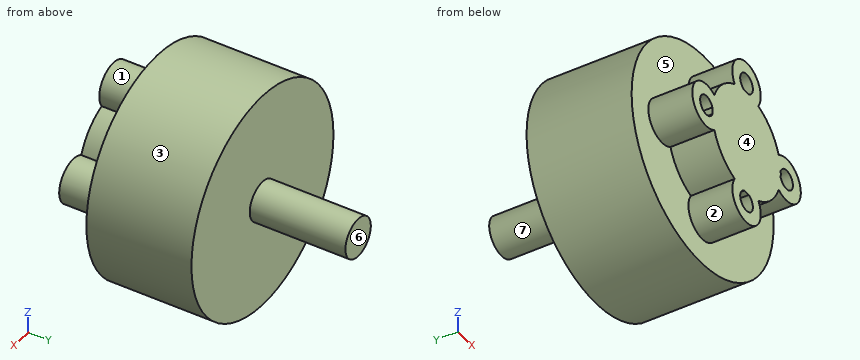
```python
from build123d import *

# Parameters (mm, degrees)
SKETCH1_R           = 14
BOSS_EXTRUDE1_DEPTH = 13.4
SKETCH2_R           = 2.5
BOSS_EXTRUDE2_DEPTH = 12.2
SKETCH3_R           = 6.75
BOSS_EXTRUDE3_DEPTH = 5.6


with BuildPart() as part:
    # Sketch1 → Boss-Extrude1 (new body)
    with BuildSketch(Plane(origin=(0, 0, 0), x_dir=(1, 0, 0), z_dir=(0, 1, 0))):
        Circle(SKETCH1_R)
    extrude(amount=BOSS_EXTRUDE1_DEPTH)

    # Sketch2 → Boss-Extrude2 (add)
    with BuildSketch(Plane(origin=(0, 13.4, 0), x_dir=(1, 0, 0), z_dir=(0, 1, 0))):
        Circle(SKETCH2_R)
    extrude(amount=BOSS_EXTRUDE2_DEPTH)

    # Sketch3 → Boss-Extrude3 (add)
    with BuildSketch(Plane.XZ):
        Circle(SKETCH3_R)
        with BuildLine():
            ThreePointArc((-6.734810127, 0.452584311), (-6.602756441, 1.402179513), (-6.3375, 2.323487411))
            ThreePointArc((-6.3375, 2.323487411), (-10.7, 0), (-6.3375, -2.323487411))
            ThreePointArc((-6.3375, -2.323487411), (-6.602756441, -1.402179513), (-6.734810127, -0.452584311))
            ThreePointArc((-6.734810127, -0.452584311), (-9.15, 0), (-6.734810127, 0.452584311))
        make_face()
        with BuildLine():
            ThreePointArc((0.452584311, 6.734810127), (1.402179513, 6.602756441), (2.323487411, 6.3375))
            ThreePointArc((2.323487411, 6.3375), (0, 10.7), (-2.323487411, 6.3375))
            ThreePointArc((-2.323487411, 6.3375), (-1.402179513, 6.602756441), (-0.452584311, 6.734810127))
            ThreePointArc((-0.452584311, 6.734810127), (0, 9.15), (0.452584311, 6.734810127))
        make_face()
        with BuildLine():
            ThreePointArc((-2.323487411, -6.3375), (0, -10.7), (2.323487411, -6.3375))
            ThreePointArc((2.323487411, -6.3375), (1.402179513, -6.602756441), (0.452584311, -6.734810127))
            ThreePointArc((0.452584311, -6.734810127), (0, -9.15), (-0.452584311, -6.734810127))
            ThreePointArc((-0.452584311, -6.734810127), (-1.402179513, -6.602756441), (-2.323487411, -6.3375))
        make_face()
        with BuildLine():
            ThreePointArc((6.3375, 2.323487411), (6.602756441, 1.402179513), (6.734810127, 0.452584311))
            ThreePointArc((6.734810127, 0.452584311), (9.15, 0), (6.734810127, -0.452584311))
            ThreePointArc((6.734810127, -0.452584311), (6.602756441, -1.402179513), (6.3375, -2.323487411))
            ThreePointArc((6.3375, -2.323487411), (10.7, 0), (6.3375, 2.323487411))
        make_face()
    extrude(amount=BOSS_EXTRUDE3_DEPTH)


solid = part.part
```
Can you work these out from the model? Positions are in its coordinate system, mm. Face numbers are marked on the shaded views. A direction names the side the tool comes from. Coordinates: 2 decimals unless noted, no trailing zeros. Write each loop counter-clockwise with the first axis right and the second up, starting at its lowest first coordinate (ties: lowest second). Pieces come first, ordered by that corner, then holes. Notation, with made-up numbers: M -20.75,43 L 13.25,43 A14 cw 13.25,48 Z; hole C 39.25,8.5 d1. An arc over 180 degrees is marked long. Write item = value, one per line. Start each with the question number.
Q1. If we section it at B-B, the plane x = 0: Write out the boundary of the cut face in (y, z).
Q2. If I drill on L1, parallel to X at y = -3.05, z = 0; L2, parallel to X at y = -2.95, z = 7.9, over which ranges is the centre line in solid material (lowest first)? Write a range as [from, to].
Q3. On a 3-axis mill with a long thin cutter (end or side, diameter ignored), from which of +Z, -Z, +X, -X, +Y, -Y can I reach the whole of each face in a straight line? I mean the marked faces 5, 6 and 7. Say none if no direction works.
Q4. If we section it at A-A, the plane z = 0: Write out the boundary of the cut face in (x, y), then the cut area to 3 significant figures.
Q5. Thinking about a two-plate mould opening in Z: for the marked faces 1, 2, 3 and 4, which applies, released by +Z, released by -Z, zero draft, split by the parting line, or undercut?
Q6. I'm going to push flat-ended pins straight in: pin 1 (12 mm diameter, centred on x = 1, z = -10, fed in from +Y); pin 2 (1 mm diameter, centred on x = 7.5, y = 2, fed in from +Z); pin 3 (1.5 mm diameter, centred on x = 7.9, z = 0, fed in from -Y). Where does each tip first touch, or does it pass through?
Q7. If we section it at D-D, the plane z = 7.9: Write out the boundary of the cut face in (x, y), then the cut area to 3 significant figures.
Q8. If we section it at C-C, the plane y = 2: Write out the boundary of the cut face in (x, z).
Check sheet entries:
q1.outline = M -5.6,-10.7 L 0,-10.7 L 0,-14 L 13.4,-14 L 13.4,-2.5 L 25.6,-2.5 L 25.6,2.5 L 13.4,2.5 L 13.4,14 L 0,14 L 0,10.7 L -5.6,10.7 L -5.6,9.15 L 0,9.15 L 0,6.75 L -5.6,6.75 L -5.6,-6.75 L 0,-6.75 L 0,-9.15 L -5.6,-9.15 Z
q2.L1 = [-10.7, -9.15], [-6.75, 6.75], [9.15, 10.7]
q2.L2 = [-2.8, -1.25], [1.25, 2.8]
q3.face_5 = -Y
q3.face_6 = +Z, -Z, +X, -X, +Y
q3.face_7 = +Y
q4.outline = M -14,0 L -10.7,0 L -10.7,-5.6 L -9.15,-5.6 L -9.15,0 L -6.75,0 L -6.75,-5.6 L 6.75,-5.6 L 6.75,0 L 9.15,0 L 9.15,-5.6 L 10.7,-5.6 L 10.7,0 L 14,0 L 14,13.4 L 2.5,13.4 L 2.5,25.6 L -2.5,25.6 L -2.5,13.4 L -14,13.4 Z
q4.area = 529 mm²
q5.face_1 = undercut
q5.face_2 = undercut
q5.face_3 = split by the parting line
q5.face_4 = zero draft
q6.pin_1 = 13.4
q6.pin_2 = 12.12
q6.pin_3 = 0
q7.outline = M -11.56,0 L -2.8,0 L -2.8,-5.6 L -1.25,-5.6 L -1.25,0 L 1.25,0 L 1.25,-5.6 L 2.8,-5.6 L 2.8,0 L 11.56,0 L 11.56,13.4 L -11.56,13.4 Z
q7.area = 327 mm²
q8.outline = C 0,0 d28
